from build123d import *

# Parameters (mm, degrees)
BOSS_EXTRUDE1_DEPTH       = 64
SKETCH2_W                 = 100
SKETCH2_H                 = 50
BOSS_EXTRUDE2_DEPTH       = 4
BOSS_EXTRUDE3_DEPTH       = 4
SKETCH4_W                 = 25
SKETCH4_H                 = 35
BOSS_EXTRUDE4_DEPTH       = 4
CHAMFER1_SIZE             = 10
CHAMFER2_SIZE             = 2
F_6_0MM_START             = -4
F_6_0MM_DOWEL_SLOT1_DEPTH = 4
FILLET1_R                 = 4


# Read off the part's stored shape, not the designer's step: Ø6.0mm Dowel Slot1
with BuildPart() as part:
    # Sketch1 → Boss-Extrude1 (new body)
    with BuildSketch(Plane(origin=(0, 0, 0), x_dir=(1, 0, 0), z_dir=(0, 1, 0))):
        Polygon((0, 0), (100, 0), (100, -50), (96, -50), (96, -4), (0, -4), align=None)
    extrude(amount=BOSS_EXTRUDE1_DEPTH)

    # Sketch2 → Boss-Extrude2 (add)
    with BuildSketch(Plane.XZ):
        with Locations((50, 25)):
            Rectangle(SKETCH2_W, SKETCH2_H)
    extrude(amount=BOSS_EXTRUDE2_DEPTH)

    # Sketch3 → Boss-Extrude3 (add)
    with BuildSketch(Plane(origin=(0, 64, 0), x_dir=(1, 0, 0), z_dir=(0, 1, 0))):
        Polygon((96, -4), (81, -4), (96, -19), align=None)
    extrude(amount=-BOSS_EXTRUDE3_DEPTH)

    # Sketch4 → Boss-Extrude4 (add)
    with BuildSketch(Plane.XZ.offset(4)):
        with Locations((40, -17.5)):
            Rectangle(SKETCH4_W, SKETCH4_H)
    extrude(amount=-BOSS_EXTRUDE4_DEPTH)

    # Chamfer1
    chamfer1_edges = [part.edges().sort_by_distance(p)[0] for p in [
        (52.5, -2, 0),
        (27.5, -2, 0),
    ]]
    chamfer(chamfer1_edges, length=CHAMFER1_SIZE)

    # Chamfer2
    chamfer2_edges = [part.edges().sort_by_distance(p)[0] for p in [
        (52.5, -2, -35),
        (27.5, -2, -35),
    ]]
    chamfer(chamfer2_edges, length=CHAMFER2_SIZE)

    # Ø6.0mm Dowel Slot1 outline → Ø6.0mm Dowel Slot1 (cut)
    with BuildSketch(Plane(origin=(0, 0, 0), x_dir=(1, 0, 0), z_dir=(0, 1, 0)).offset(F_6_0MM_START)):
        with BuildLine():
            Line((34.75, 6.75), (45.25, 6.75))
            ThreePointArc((45.25, 6.75), (48.5, 10), (45.25, 13.25))
            Line((45.25, 13.25), (34.75, 13.25))
            ThreePointArc((34.75, 13.25), (31.5, 10), (34.75, 6.75))
        make_face()
        with BuildLine():
            Line((34.75, 21.75), (45.25, 21.75))
            ThreePointArc((45.25, 21.75), (48.5, 25), (45.25, 28.25))
            Line((45.25, 28.25), (34.75, 28.25))
            ThreePointArc((34.75, 28.25), (31.5, 25), (34.75, 21.75))
        make_face()
    extrude(amount=F_6_0MM_DOWEL_SLOT1_DEPTH, mode=Mode.SUBTRACT)

    # Fillet1
    fillet1_edges = [part.edges().sort_by_distance(p)[0] for p in [
        (40, 0, 0),
    ]]
    fillet(fillet1_edges, radius=FILLET1_R)


solid = part.part
For this review, take the finished solid that the model builds, in its own axes (mm). A direction names the side the tool comes from. Give positions to 0.01 mm unless a question says otherwise; leave off trailing zeros. Loops run counter-clockwise (first coordinate to the right, second up) from the corner with the lowest first, then second, coordinate; pieces in that order, holes last.
Item 1: Take a section at B-B, the plane x = 84. State the section outline as (y, z) points, and give its area (3 significant figures).
Item 2: Tool access review of faces 1 (the flat face through (40, 0, -19)), 2 (the flat face through (88, 62, 11)), 3 (the flat face through (40, -2, -21.75)): name each direction out of +Z, -Z, +X, -X, +Y, -Y from which nothing blocks a thin tool from reaching the whole face with its end or side.
Item 3: For line 1 along Z through (x, y) = (85.5, 9); line 2 along X through (y, z) = (50.5, 45); line 3 along Y through (x, z) = (41.5, 41), list the stretches that pass through material, from the lowest coordinate up.
Item 4: Take a section at A-A, the plane z = -25. State the section outline as (x, y) points, and give its area (3 significant figures).
Item 5: Draft analysis for pull direction Y (two halves, no side actions). For faces 4 (the flat face through (96, 32, 27)), 5 (the flat face through (68, 64, 3)), 6 (the flat face through (52.5, -2, -22)), state which applies: +Y half, -Y half, draft (parallel to the pull), parting line (faces both ways), or undercut.
Item 6: Take a section at C-C, the plane y = 14.5. State the section outline as (x, z) points.
Item 7: Take a section at D-D, the plane y = 1.5. State the section outline as (x, z) points.
Item 8: Insertion check: pin 1 (9.5 mm diameter, centred on x = 38.5, z = -21.5, fed in from +Y); pin 2 (1 mm diameter, centred on x = 15.5, y = 54.5, fed in from -Z); pin 3 (2 mm diameter, centred on y = -1, z = -16, fed in from -X). Each pin has a flat end and moves straight along its axis. Give the tip position at first contact, or say it passes through.
Calculated:
1. outline: (-4, 0) - (64, 0) - (64, 7) - (60, 7) - (60, 4) - (0, 4) - (0, 50) - (-4, 50) - close
1. area: 468 mm2
2. face 1: -Z, +X, -X, +Y
2. face 2: +Z, -X, +Y
2. face 3: +Y, -Y
3. line 1: z = 0 to 4
3. line 2: x = 96 to 100
3. line 3: y = -4 to 0
4. outline: (27.5, -4) - (31.5, -4) - (31.5, 0) - (27.5, 0) - close; (48.5, -4) - (52.5, -4) - (52.5, 0) - (48.5, 0) - close
4. area: 32.0 mm2
5. face 4: undercut
5. face 5: +Y half
5. face 6: draft
6. outline: (0, 0) - (100, 0) - (100, 50) - (96, 50) - (96, 4) - (0, 4) - close
7. outline: (0, 0) - (17.5, 0) - (18.38, -0.88) - (61.62, -0.88) - (62.5, 0) - (100, 0) - (100, 50) - (96, 50) - (96, 4) - (0, 4) - close
8. pin 1: stops at y = 0
8. pin 2: stops at z = 0
8. pin 3: stops at x = 27.5
